Geometry check sheet. Reference: the model listing, model coordinates, mm. Face numbers are marked on the shaded views. A direction names the side the tool comes from. Give positions to 0.01 mm unless a question says otherwise; leave off trailing zeros. Use a Markdown table: item, result. Add a question column.
1. Set-up check for the marked faces 1, 2 and 3: record each of +Z, -Z, +X, -X, +Y, -Y from which the full face is reachable in a straight line by a thin tool's end or side.
2. Material ranges on L1, parallel to Z at x = -21, y = 14.75; L2, parallel to X at y = 12, z = 12.5; L3, parallel to X at y = 11, z = -1, recorded low to high.
3. Draft check along X on the marked faces 4, 5 and 6. Enter one of: pulls with the +X half, pulls with the -X half, needs draft (parallel to the pull), parting line crosses it, or undercut.
4. Depth check by flat-ended pin: P1, Ø10, axis at y = 5.5, z = -16, coming from the -X side; P2, Ø5, axis at x = 5, y = 14.5, coming from the +Z side; P3, Ø1.5, axis at x = 0, z = -9, coming from the -Y side; P4, Ø5, axis at y = 16, z = 2, coming from the -X side. Enter the tip coordinate at first touch or a pass-through.
5. Cross-section at A-A on x = 0. Count the separate pieces of the cut face and the enclosed holes in it, and give its area (3 significant figures).
from build123d import *

# Parameters (mm, degrees)
SKETCH_1_R          = 32
SKETCH_1_R_2        = 4
SKETCH_1_R_3        = 3
EXTRUDE_1_DEPTH     = 19
FILLET_1_R          = 2
SKETCH_2_R          = 5.375
CUT_EXTRUDE_1_DEPTH = 15.5
SKETCH_3_R          = 2.625
CUT_EXTRUDE_2_DEPTH = 15
SKETCH_4_R          = 1.75
CUT_EXTRUDE_3_DEPTH = 50.081564832
SKETCH_5_R          = 1.25
CUT_EXTRUDE_4_DEPTH = 50.081564832
SKETCH_6_R          = 3
CUT_EXTRUDE_5_DEPTH = 8
SKETCH_7_R          = 1.95
CUT_EXTRUDE_6_DEPTH = 3
CHAMFER_1_SIZE      = 1
SKETCH_8_R          = 0.75
CUT_EXTRUDE_7_DEPTH = 50.081564832


with BuildPart() as part:
    # Эскиз1 → Бобышка-Вытянуть1 (new body)
    with BuildSketch(Plane(origin=(0, 0, 0), x_dir=(1, 0, 0), z_dir=(0, 1, 0))):
        with Locations(Location((0, 0, 0), (0, 0, 270))):
            Circle(SKETCH_1_R)
        with Locations(Location((0, 0, 0), (0, 0, 270))):
            Circle(SKETCH_1_R_2, mode=Mode.SUBTRACT)
        with Locations(Location((0, 25, 0), (0, 0, 270))):
            Circle(SKETCH_1_R_3, mode=Mode.SUBTRACT)
        with Locations(Location((21.650635095, -12.5, 0), (0, 0, 270))):
            Circle(SKETCH_1_R_3, mode=Mode.SUBTRACT)
        with Locations(Location((-21.650635095, -12.5, 0), (0, 0, 270))):
            Circle(SKETCH_1_R_3, mode=Mode.SUBTRACT)
    extrude(amount=EXTRUDE_1_DEPTH)

    # Скругление1
    fillet_1_edges = [part.edges().sort_by_distance(p)[0] for p in [
        (0, 0, -32),
    ]]
    fillet(fillet_1_edges, radius=FILLET_1_R)

    # Эскиз2 → Вырез-Вытянуть1 (cut)
    with BuildSketch(Plane(origin=(0, 19, 0), x_dir=(1, 0, 0), z_dir=(0, 1, 0))):
        with Locations(Location((0, 25, 0), (0, 0, 270))):
            Circle(SKETCH_2_R)
        with Locations(Location((21.650635095, -12.5, 0), (0, 0, 270))):
            Circle(SKETCH_2_R)
        with Locations(Location((-21.650635095, -12.5, 0), (0, 0, 270))):
            Circle(SKETCH_2_R)
    extrude(amount=-CUT_EXTRUDE_1_DEPTH, mode=Mode.SUBTRACT)

    # Эскиз3 → Вырез-Вытянуть2 (cut)
    with BuildSketch(Plane.XZ):
        with Locations(Location((0, 25, 0), (0, 0, 270))):
            Circle(SKETCH_3_R)
        with Locations(Location((21.650635095, -12.5, 0), (0, 0, 270))):
            Circle(SKETCH_3_R)
        with Locations(Location((-21.650635095, -12.5, 0), (0, 0, 270))):
            Circle(SKETCH_3_R)
    extrude(amount=-CUT_EXTRUDE_2_DEPTH, mode=Mode.SUBTRACT)

    # Эскиз4 → Вырез-Вытянуть3 (cut, through all)
    with BuildSketch(Plane.XZ):
        with Locations(Location((0, 14, 0), (0, 0, 270))):
            Circle(SKETCH_4_R)
        with Locations(Location((14, 0, 0), (0, 0, 270))):
            Circle(SKETCH_4_R)
        with Locations(Location((0, -14, 0), (0, 0, 270))):
            Circle(SKETCH_4_R)
        with Locations(Location((-14, 0, 0), (0, 0, 270))):
            Circle(SKETCH_4_R)
    extrude(amount=-CUT_EXTRUDE_3_DEPTH, mode=Mode.SUBTRACT)

    # Эскиз5 → Вырез-Вытянуть4 (cut, through all)
    with BuildSketch(Plane(origin=(0, 19, 0), x_dir=(1, 0, 0), z_dir=(0, 1, 0))):
        with Locations(Location((0, 9, 0), (0, 0, 270))):
            Circle(SKETCH_5_R)
        with Locations(Location((7.794228634, -4.5, 0), (0, 0, 270))):
            Circle(SKETCH_5_R)
        with Locations(Location((-7.794228634, -4.5, 0), (0, 0, 270))):
            Circle(SKETCH_5_R)
    extrude(amount=-CUT_EXTRUDE_4_DEPTH, mode=Mode.SUBTRACT)

    # Эскиз6 → Вырез-Вытянуть5 (cut)
    with BuildSketch(Plane.XZ):
        with Locations(Location((0, 14, 0), (0, 0, 270))):
            Circle(SKETCH_6_R)
        with Locations(Location((14, 0, 0), (0, 0, 270))):
            Circle(SKETCH_6_R)
        with Locations(Location((0, -14, 0), (0, 0, 270))):
            Circle(SKETCH_6_R)
        with Locations(Location((-14, 0, 0), (0, 0, 270))):
            Circle(SKETCH_6_R)
    extrude(amount=-CUT_EXTRUDE_5_DEPTH, mode=Mode.SUBTRACT)

    # Эскиз7 → Вырез-Вытянуть6 (cut)
    with BuildSketch(Plane.XZ):
        with Locations(Location((7.794228634, 4.5, 0), (0, 0, 270))):
            Circle(SKETCH_7_R)
        with Locations(Location((0, -9, 0), (0, 0, 270))):
            Circle(SKETCH_7_R)
        with Locations(Location((-7.794228634, 4.5, 0), (0, 0, 270))):
            Circle(SKETCH_7_R)
    extrude(amount=-CUT_EXTRUDE_6_DEPTH, mode=Mode.SUBTRACT)

    # Фаска1
    chamfer_1_edges = [part.edges().sort_by_distance(p)[0] for p in [
        (21.650635095, 0, 9.5),
        (-21.650635095, 0, 9.5),
        (0, 0, 27.625),
        (21.650635095, 0, -9.875),
        (-21.650635095, 0, -9.875),
        (0, 0, -4),
        (0, 0, -28),
    ]]
    chamfer(chamfer_1_edges, length=CHAMFER_1_SIZE)

    # Эскиз8 → Вырез-Вытянуть7 (cut, through all)
    with BuildSketch(Plane.XZ):
        with Locations(Location((-8, 23.685438565, 0), (0, 0, 270))):
            Circle(SKETCH_8_R)
        with Locations(Location((8, 23.685438565, 0), (0, 0, 270))):
            Circle(SKETCH_8_R)
        with Locations(Location((24.512191497, -4.914516052, 0), (0, 0, 270))):
            Circle(SKETCH_8_R)
        with Locations(Location((16.512191497, -18.770922513, 0), (0, 0, 270))):
            Circle(SKETCH_8_R)
        with Locations(Location((-16.512191497, -18.770922513, 0), (0, 0, 270))):
            Circle(SKETCH_8_R)
        with Locations(Location((-24.512191497, -4.914516052, 0), (0, 0, 270))):
            Circle(SKETCH_8_R)
    extrude(amount=-CUT_EXTRUDE_7_DEPTH, mode=Mode.SUBTRACT)


solid = part.part
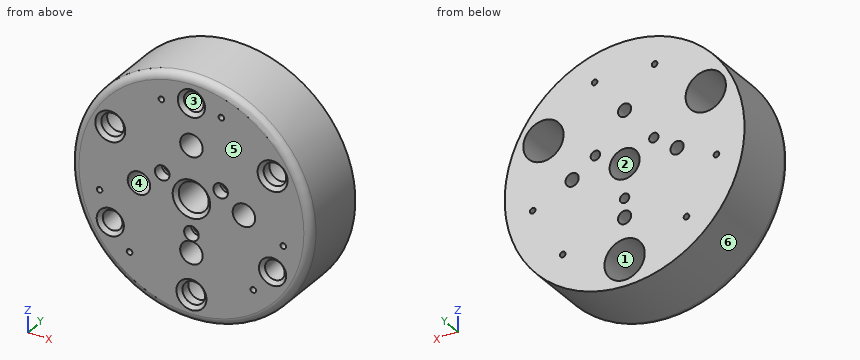
Values found:
| question | item | result |
|---|---|---|
| 1 | face 1 | +Y |
| 1 | face 2 | +Y, -Y |
| 1 | face 3 | -Y |
| 2 | L1 | z = -24.15 to -15.04, -9.96 to 7.16, 17.84 to 24.15 |
| 2 | L2 | x = -29.46 to -27.03, -16.28 to -0.9, 0.9 to 16.28, 27.03 to 29.46 |
| 2 | L3 | x = -31.98 to -15.44, -12.56 to -3.87, 3.87 to 12.56, 15.44 to 31.98 |
| 3 | face 4 | undercut |
| 3 | face 5 | needs draft |
| 3 | face 6 | parting line crosses it |
| 4 | P1 | stops at x = -30.05 |
| 4 | P2 | stops at z = 31.9 |
| 4 | P3 | passes through |
| 4 | P4 | stops at x = -32 |
| 5 | separate pieces | 6 |
| 5 | enclosed holes | 0 |
| 5 | area | 568 mm2 |
